Model file for the job. Use its own axes, mm. A direction names the side the tool comes from. Round coordinates to 2 decimals unless told otherwise and drop trailing zeros. Order: outer loops, then holes, each group sorted by start corner. A loop starts at its lowest first (then second) coordinate and runs counter-clockwise, first axis right, second up. Notation, with made-up numbers: (20.5, 0.5) - (35.5, 0.5) arc R29 cw to (35.5, 38.5) - close; hole circle Ø9 at (13, -21). An arc over 180 degrees is marked (long way). Put each result on its own line as item: value. Start each with the question number.
Item 1: Which spindle directions (+Z, -Z, +X, -X, +Y, -Y) get a long thin tool onto all of the face, cutting with end or side? Do faces 1 (the face through (-10, 27, 0)), 2 (the face through (10, 2, 17)). Say none if no direction does.
Item 2: Saw through at B-B on x = -107.5. List the corners of the cut face in (y, z).
Item 3: Probe probe 1 along Y at (x, z) = (333, 28.25); probe 2 along Z at (x, y) = (-173.5, 3.5). List the from-to ranges inside material, lowest first.
Item 4: Pin check, flat tips, straight feed: pin 1 Ø1 at (y, z) = (37.5, 1.5) entering from -X; pin 2 Ø0.6 at (y, z) = (38.5, 1.5) entering from -X; pin 3 Ø0.6 at (y, z) = (37, 1) entering from +X; pin 4 Ø8 at (y, z) = (19, 9) entering from -X (3 decimals). Stop position of each tip, or through.
Item 5: Saw through at C-C on z = 9.25. List the corners of the cut face in (x, y).
Item 6: Saw through at A-A on y = 40. List the corners of the cut face in (x, z).
Autodesk Inventor part; units mm, degrees
ref_plane "YZ Plane" through (0, 0, 0) normal (1, 0, 0) x (0, 1, 0)
ref_plane "XZ Plane" through (0, 0, 0) normal (0, 1, 0) x (-1, 0, 0)
ref_plane "XY Plane" through (0, 0, 0) normal (0, 0, 1) x (1, 0, 0)
sketch "Sketch1" plane through (0, 0, 0) normal (0, 0, 1) x (1, 0, 0)
  line L0 (-750, 48.2006) -> (750, 48.2006)
  line L1 (750, 48.2006) -> (750, 0)
  line L2 (750, 0) -> (-750, 0)
  line L3 (-750, 0) -> (-750, 48.2006)
  point P0 (0, 0)
  point P1 (0, 0)
  dimension "d0" = 1500
  dimension "d1" = 48.2006
extrude "Plate1" add sketch "Sketch1" along normal blind 2
sketch "Sketch2" plane through (750, 2, 0) normal (0, -1, 0) x (1, 0, 0)
  line L0 (-1500, 0) -> (0, 0)
  line L1 (0, 0) -> (0, 30)
  line L2 (0, 30) -> (-1500, 30)
  line L3 (-1500, 30) -> (-1500, 0)
edge flange "Flange1" height 30 angle 90 thickness 2 bend radius 2.75 thickness toward (0, -1, 0) relief round relief width 2 relief depth 1 edges at (0, 0, 2) wall of the first edge with corners at (-750, 2, 0) (750, 2, 0) (750, 2, 30) (-750, 2, 30)
bend "Bend1"
corner "Corner1"
sketch "Sketch5" plane through (0, 0, 0) normal (0, 0, -1) x (-1, 0, 0)
  line L0 (750, 48.2006) -> (-750, 48.2006)
  line L1 (-1, 30) -> (-1, 48.2006)
  line L2 (750, 0) -> (-750, 0)
  line L3 (-1, 30) -> (1, 30)
  line L4 (1, 30) -> (1, 48.2006)
  point P0 (0, 0)
  point P1 (0, 30)
  point P2 (0, 0)
  dimension "d27" = 2
  dimension "d28" = 30
extrude "Extrusion1" cut sketch "Sketch5" against normal through all
pattern_linear "Rectangular Pattern1" count 3 spacing 500 along (1, 0, 0) of "Extrusion1" first direction both ways yes
sketch "Sketch6" plane through (0, 0, 0) normal (0, 0, -1) x (-1, 0, 0)
  line L0 (-750, 48.2006) -> (-750, 4.75)
  circle A0 centre (-750, 48.2006) radius 22.5
  line L1 (-750, 48.2006) -> (750, 48.2006)
  line L2 (-1, 48.2006) -> (-1, 30)
  line L3 (-499, 48.2006) -> (-499, 30)
  line L4 (-1, 30) -> (-499, 30) construction
  circle A1 centre (-250, 48.2006) radius 22.5
  point P0 (0, 0)
  point P1 (-727.5, 48.2006)
  point P2 (-750, 25.7006)
  point P3 (-250, 30)
  dimension "d24" = 45
extrude "Extrusion2" cut sketch "Sketch6" along normal mid plane 30 contours L1 A0 L0 | A1 L1 | L1 A1 picked at (-748.3311, 33.3886)
mirror "Mirror1" about plane through (0, 0, 0) normal (1, 0, 0) of "Extrusion2"
sketch "Sketch7" plane through (0, 0, 2) normal (0, 0, 1) x (1, 0, 0)
  arc A0 (-750, 25.7006) -> (-727.5, 48.2006) centre (-750, 48.2006) ccw
  line L0 (-750, 4.75) -> (-750, 25.7006)
  line L1 (-750, 4.75) -> (750, 4.75)
  line L2 (750, 25.7006) -> (750, 4.75)
  arc A1 (727.5, 48.2006) -> (750, 25.7006) centre (750, 48.2006) ccw
  line L3 (501, 48.2006) -> (727.5, 48.2006)
  line L4 (501, 48.2006) -> (501, 30)
  line L5 (501, 30) -> (499, 30)
  line L6 (499, 30) -> (499, 48.2006)
  line L7 (1, 48.2006) -> (227.5, 48.2006)
  line L8 (1, 48.2006) -> (1, 30)
  line L9 (1, 30) -> (-1, 30)
  line L10 (-1, 30) -> (-1, 48.2006)
  line L11 (-499, 48.2006) -> (-272.5, 48.2006)
  line L12 (-499, 48.2006) -> (-499, 30)
  line L13 (-499, 30) -> (-501, 30)
  line L14 (-501, 30) -> (-501, 48.2006)
  line L15 (-727.5, 48.2006) -> (-501, 48.2006)
  line L16 (650, 4.75) -> (650, 48.2006) construction
  line L17 (-750, 4.75) -> (750, 4.75)
  circle A2 centre (650, 26.4753) radius 5
  circle A3 centre (630, 26.4753) radius 5
  line L18 (272.5, 48.2006) -> (499, 48.2006)
  arc A4 (227.5, 48.2006) -> (272.5, 48.2006) centre (250, 48.2006) ccw
  line L19 (-227.5, 48.2006) -> (-1, 48.2006)
  arc A5 (-272.5, 48.2006) -> (-227.5, 48.2006) centre (-250, 48.2006) ccw
  point P0 (0, 0)
  dimension "d29" = 100
  dimension "d30" = 10
  dimension "d31" = 10
  dimension "d32" = 20
extrude "Extrusion3" [suppressed]
mirror "Mirror2" [suppressed]
sketch "Sketch8" plane through (0, 0, 2) normal (0, 0, 1) x (1, 0, 0)
  line L0 (494, 43.2006) -> (494, 31.2006) construction
  line L1 (494, 31.2006) -> (294, 31.2006) construction
  line L2 (294, 31.2006) -> (294, 43.2006) construction
  line L3 (294, 43.2006) -> (494, 43.2006) construction
  line L4 (501, 48.2006) -> (727.5, 48.2006)
  line L5 (272.5, 48.2006) -> (499, 48.2006)
  point P0 (0, 0)
  dimension "d35" = 200
  dimension "d36" = 12
  dimension "d39" = 5
  dimension "d40" = 5
mark "Mark1"
equation "\"d1\" = Стрингер_4"
equation "\"d27\" = d18"
equation "\"d2\" = Thickness"
equation "\"d3\" = BendReliefWidth"
equation "\"d4\" = BendReliefDepth"
equation "\"d5\" = MinimumRemnant"
equation "\"d6\" = TransitionRadius"
equation "\"d9\" = BendRadius"
equation "\"d10\" = CornerReliefSize"
equation "\"d11\" = GapSize"
equation "\"d12\" = JacobiRadiusSize"
equation "\"BendReliefWidth\" = Thickness"
equation "\"BendReliefDepth\" = 0.5 * Thickness"
equation "\"CornerReliefSize\" = 4 * Thickness"
equation "\"MinimumRemnant\" = 2 * Thickness"
equation "\"TransitionRadius\" = BendRadius"
equation "\"JacobiRadiusSize\" = BendRadius"
equation "\"GapSize\" = Thickness"
equation "\"d18\" = Thickness"
properties part number "MSC 064 stringer board ##" material "Stainless Steel"
Results found:
1. face 1: -Z, +X, -X, +Y, -Y
1. face 2: +Z, +X, -X, +Y
2. outline: (0, 4.75) arc R4.75 ccw to (4.75, 0) - (48.2, 0) - (48.2, 2) - (4.75, 2) arc R2.75 cw to (2, 4.75) - (2, 30) - (0, 30) - close
3. probe 1: y = 0 to 2
3. probe 2: z = 0.17 to 2.3
4. pin 1: stops at x = -730.49
4. pin 2: stops at x = -729.84
4. pin 3: stops at x = 730.66
4. pin 4: passes through
5. outline: (-750, 0) - (750, 0) - (750, 2) - (-750, 2) - close
6. outline: (-729.05, 0) - (-501, 0) - (-501, 2) - (-729.05, 2) - close; (-499, 0) - (-270.95, 0) - (-270.95, 2) - (-499, 2) - close; (-229.05, 0) - (-1, 0) - (-1, 2) - (-229.05, 2) - close; (1, 0) - (229.05, 0) - (229.05, 2) - (1, 2) - close; (270.95, 0) - (499, 0) - (499, 2) - (270.95, 2) - close; (501, 0) - (729.05, 0) - (729.05, 2) - (501, 2) - close
